Autodesk Inventor part; units mm, degrees
ref_plane "YZ Plane" through (0, 0, 0) normal (1, 0, 0) x (0, 1, 0)
ref_plane "XZ Plane" through (0, 0, 0) normal (0, 1, 0) x (-1, 0, 0)
ref_plane "XY Plane" through (0, 0, 0) normal (0, 0, 1) x (1, 0, 0)
sketch "Sketch1" plane through (0, 0, 0) normal (1, 0, 0) x (0, 1, 0)
  circle A0 centre (0, 0) radius 3.5
  dimension "d0" = 7
extrude "Extrusion1" add sketch "Sketch1" along normal blind 29
sketch "Sketch2" plane through (29, 0, 0) normal (1, 0, 0) x (0, 0, -1)
  line L0 (-5, -1.5) -> (5, -1.5)
  line L1 (5, -1.5) -> (5, 1.5)
  line L2 (5, 1.5) -> (-5, 1.5)
  line L3 (-5, 1.5) -> (-5, -1.5)
  line L4 (-5, -1.5) -> (5, 1.5) construction
  line L5 (5, -1.5) -> (-5, 1.5) construction
  point P0 (0, 0)
  dimension "d3" = 10
  dimension "d4" = 3
extrude "Extrusion2" cut sketch "Sketch2" against normal blind 8
sketch "Sketch3" plane through (0, 0, 0) normal (-1, 0, 0) x (0, 0, 1)
  circle A0 centre (0, 0) radius 1.5
  dimension "d7" = 3
extrude "Extrusion3" add sketch "Sketch3" along normal blind 26
sketch "Sketch4" plane through (-26, 0, 0) normal (-1, 0, 0) x (0, 0, 1)
  circle A0 centre (0, 0) radius 2.5
  dimension "d10" = 5
extrude "Extrusion4" add sketch "Sketch4" against normal blind 5
properties part number "solenoid piston"
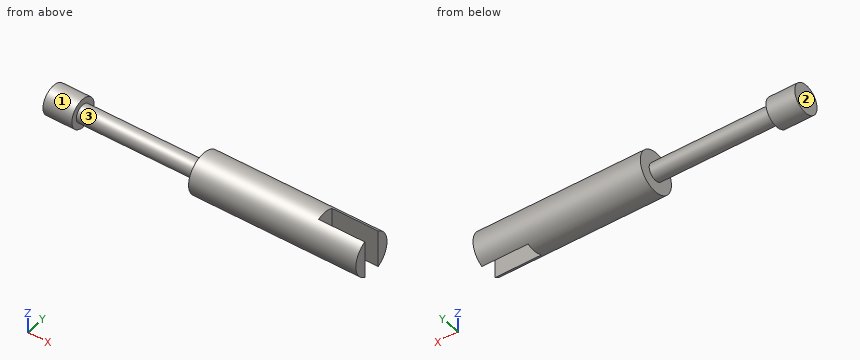
Input: part model. Units: mm. Frame: model coordinates. Face numbers are marked on the shaded views. A direction names the side the tool comes from. Coordinates: 2 decimals unless noted, no trailing zeros. Order: outer loops, then holes, each group sorted by start corner. A loop starts at its lowest first (then second) coordinate and runs counter-clockwise, first axis right, second up. Notation, with made-up numbers: (84, -6) - (106, -6) arc R32 ccw to (106, 29) - close; hole circle Ø3 at (71.5, 51). An arc over 180 degrees is marked (long way). Return JSON: item names as keys, results as strings.
Q1. Cut plane B-B (z = 0). Return loops of the section in (x, y), then the cut area to 3 significant figures.
The answers:
{"outline": "(-26, -2.5) - (-21, -2.5) - (-21, -1.5) - (0, -1.5) - (0, -3.5) - (29, -3.5) - (29, -1.5) - (21, -1.5) - (21, 1.5) - (29, 1.5) - (29, 3.5) - (0, 3.5) - (0, 1.5) - (-21, 1.5) - (-21, 2.5) - (-26, 2.5) - close", "area": "267 mm2"}
Q2. Cut plane C-C (x = 26). Return loops of the section in (y, z), then the cut area to 3 significant figures.
The answers:
{"outline": "(-1.5, -3.16) - (-1.5, 3.16) arc R3.5 ccw to start; (1.5, -3.16) arc R3.5 ccw to (1.5, 3.16) - close", "area": "18.1 mm2"}
Q3. Cut plane D-D (x = 1). Return loops of the section in (y, z), then the cut area to 3 significant figures.
The answers:
{"outline": "circle Ø7 at (0, 0)", "area": "38.5 mm2"}
Q4. Cut plane A-A (y = 0). Return loops of the section in (x, z), then the cut area to 3 significant figures.
The answers:
{"outline": "(-26, -2.5) - (-21, -2.5) - (-21, -1.5) - (0, -1.5) - (0, -3.5) - (21, -3.5) - (21, 3.5) - (0, 3.5) - (0, 1.5) - (-21, 1.5) - (-21, 2.5) - (-26, 2.5) - close", "area": "235 mm2"}
Q5. First-contact query: pin 1 (1.5 mm diameter, centred on x = 10, y = -1.5, fed in from +Z); pin 2 (1 mm diameter, centred on x = -10, z = -1.5, fed in from +Y). Flat tips, straight axial feed; report the tip coordinate or a pass-through.
The answers:
{"pin 1": "stops at z = 3.42", "pin 2": "stops at y = 1.12"}
Q6. Ray query, probe 1 along X at (y, z) = (-0.75, 1.5); probe 2 along X at (y, z) = (-2.25, 0); probe 3 along Y at (x, z) = (26.5, 1). Return the intervals inside material, ascending.
The answers:
{"probe 1": "x = -26 to -21, 0 to 21", "probe 2": "x = -26 to -21, 0 to 29", "probe 3": "y = -3.35 to -1.5, 1.5 to 3.35"}
Q7. Access query for the marked faces 1, 2 and 3. Directions: +Z, -Z, +X, -X, +Y, -Y. A direction counts if a zero-diameter tool reaches every point of the face in a straight line with its end or side. Return the directions, or none.
The answers:
{"face 1": "-X", "face 2": "+Z, -Z, -X, +Y, -Y", "face 3": "none"}
